For this review, take the finished solid that the model builds, in its own axes (mm). A direction names the side the tool comes from. Give positions to 0.01 mm unless a question says otherwise; leave off trailing zeros. Write each loop counter-clockwise with the first axis right and the second up, starting at its lowest first coordinate (ties: lowest second). Pieces come first, ordered by that corner, then holes. Notation, with made-up numbers: M 19,34 L 50,34 A23 ccw 50,46 Z; hole C -5,-25.5 d11. An arc over 180 degrees is marked long. One line per item, written item: value. Start each with the question number.
Item 1: Mouldability with a two-part tool opening along Y and no side actions: class faces 5 (the face through (-40, -36, 8)), 6 (the face through (-76, 30, 66)), 7 (the face through (17, 13, 16)) as released by +Y, released by -Y, zero draft, split by the parting line, or undercut.
Item 2: Clearance check with flat-ended pins moving along their axes: pin 1 Ø6 at (x, y) = (-19.5, 52.5) entering from +Z; pin 2 Ø12 at (y, z) = (-33, 98) entering from -X; pin 3 Ø3 at (x, z) = (-45, 83) entering from +Y. State where each tip first meets the part, or that it passes through.
Item 3: Consider section B-B, the plane y = 0. Give the number of separate pieces and of enclosed holes in the cut face, and give its area (3 significant figures).
Item 4: To check wall thickness, follow probe 1 along X at (y, z) = (-31, 11.5); probe 2 along Z at (x, y) = (0, 31); probe 3 along X at (y, z) = (46.5, 40). State the ranges of each line that lie inside material, in increasing order.
Item 5: Consider section A-A, the plane z = 8. Write out the cut boundary in (x, y).
Item 6: Tool access review of faces 1 (the face through (-40, 36, 8)), 2 (the face through (-50, 54, 66)), 3 (the face through (-76, -30, 66)), 4 (the face through (-73, 0, 76)): name each direction out of +Z, -Z, +X, -X, +Y, -Y from which nothing blocks a thin tool from reaching the whole face with its end or side.
```python
from build123d import *

# Parameters (mm, degrees)
F0_W      = 160
F0_H      = 112
F1_DEPTH  = 40
F2_W      = 80
F2_H      = 16
F3_DEPTH  = 112
F4_W      = 32
F4_H      = 16
F5_DEPTH  = 160
F6_W      = 100
F6_H      = 112
F7_DEPTH  = 36
F8_W      = 30
F8_H      = 60
F9_DEPTH  = 36
F10_W     = 30
F10_H     = 60
F11_DEPTH = 36
F15_W     = 100
F15_H     = 80
F13_W     = 160
F13_H     = 112
F17_R     = 20
F18_DEPTH = 120
F19_R     = 15
F20_DEPTH = 160
F21_R     = 15
F22_DEPTH = 112


with BuildPart() as f1:
    # F0 (on Top) → F1 (new body)
    with BuildSketch(Plane.XY):
        Rectangle(F0_W, F0_H)
    extrude(amount=F1_DEPTH)

    # F2 (on face) → F3 (cut)
    with BuildSketch(Plane.XZ.offset(56)):
        with Locations((0, 8)):
            Rectangle(F2_W, F2_H)
    extrude(amount=-F3_DEPTH, mode=Mode.SUBTRACT)

    # F4 (on face) → F5 (cut)
    with BuildSketch(Plane(origin=(-80, 0, 0), x_dir=(0, -1, 0), z_dir=(-1, 0, 0))):
        with Locations((0, 8)):
            Rectangle(F4_W, F4_H)
    extrude(amount=-F5_DEPTH, mode=Mode.SUBTRACT)

    # F6 (on face) → F7 (join)
    with BuildSketch(Plane.XY.offset(40)):
        Rectangle(F6_W, F6_H)
    extrude(amount=F7_DEPTH)

    # F8 (on face) → F9 (join)
    with BuildSketch(Plane.XY.offset(40)):
        with Locations((65, 0)):
            Rectangle(F8_W, F8_H)
    extrude(amount=F9_DEPTH)

    # F10 (on face) → F11 (join)
    with BuildSketch(Plane.XY.offset(40)):
        with Locations((-65, 0)):
            Rectangle(F10_W, F10_H)
    extrude(amount=F11_DEPTH)

    # F15 (on offset) → F16 section 0
    with BuildSketch(Plane.XY.offset(120)):
        Rectangle(F15_W, F15_H)
    # F13 (on offset) → F16 section 1
    with BuildSketch(Plane.XY.offset(40)):
        Rectangle(F13_W, F13_H)
    loft()

    # F17 (on offset) → F18 (cut)
    with BuildSketch(Plane.XY.offset(120)):
        Circle(F17_R)
    extrude(amount=-F18_DEPTH, mode=Mode.SUBTRACT)

    # F19 (on face) → F20 (cut)
    with BuildSketch(Plane.YZ.offset(80)):
        with Locations((0, 42.966103)):
            Circle(F19_R)
    extrude(amount=-F20_DEPTH, mode=Mode.SUBTRACT)

    # F21 (on face) → F22 (cut)
    with BuildSketch(Plane.XZ.offset(56)):
        with Locations((0, 39.809708)):
            Circle(F21_R)
    extrude(amount=-F22_DEPTH, mode=Mode.SUBTRACT)


solid = f1.part
```
Model answer:
1. face 5: zero draft
1. face 6: released by +Y
1. face 7: undercut
2. pin 1: stops at z = 76
2. pin 2: stops at x = -60.5
2. pin 3: stops at y = 47.7
3. separate pieces: 4
3. enclosed holes: 0
3. area: 6,970 mm2
4. probe 1: x = -80 to -40, 40 to 80
4. probe 2: z = 16 to 24.81, 54.81 to 120
4. probe 3: x = -80 to -15, 15 to 80
5. outline: M -80,-56 L -40,-56 L -40,-16 L -80,-16 Z; M -80,16 L -40,16 L -40,56 L -80,56 Z; M 40,-56 L 80,-56 L 80,-16 L 40,-16 Z; M 40,16 L 80,16 L 80,56 L 40,56 Z
6. face 1: -Z, +Y, -Y
6. face 2: +Z, -X, +Y
6. face 3: +Z, -X, -Y
6. face 4: +Z, -X, +Y, -Y
